Work out the finished part from the listing and answer in its coordinate system (mm). A direction names the side the tool comes from. Round coordinates to 2 decimals unless told otherwise and drop trailing zeros. Loops run counter-clockwise (first coordinate to the right, second up) from the corner with the lowest first, then second, coordinate; pieces in that order, holes last. Notation, with made-up numbers: (-9.75, 21.5) -> (33.25, 21.5) arc R22 cw to (33.25, 50.5) -> close; hole circle Ø1 at (60.25, 5). An arc over 180 degrees is marked (long way). Use one line per item in the form item = value.
```python
from build123d import *

# Parameters (mm, degrees)
BOSS_EXTRUDE1_DEPTH = 15
BOSS_EXTRUDE2_REACH = 43.075
SKETCH3_R           = 3.25
CUT_EXTRUDE1_DEPTH  = 42.075053256
FILLET1_R           = 1
FILLET2_R           = 1


with BuildPart() as part:
    # Sketch1 → Boss-Extrude1 (new, symmetric)
    with BuildSketch(Plane.XY):
        with BuildLine():
            Line((-22.5, 0), (-35, 0))
            Line((-35, 0), (-35, 3))
            Line((-35, 3), (-25.322914524, 3))
            ThreePointArc((-25.322914524, 3), (0, 25.5), (25.322914524, 3))
            Line((25.322914524, 3), (35, 3))
            Line((35, 3), (35, 0))
            Line((35, 0), (22.5, 0))
            ThreePointArc((22.5, 0), (0, 22.5), (-22.5, 0))
        make_face()
    extrude(amount=BOSS_EXTRUDE1_DEPTH, both=True)

    # Sketch2 → Boss-Extrude2 (add, up to next)
    with BuildSketch(Plane(origin=(0, 15.4, 0), x_dir=(1, 0, 0), z_dir=(0, 1, 0)), mode=Mode.PRIVATE) as boss_extrude2_sk1:
        with BuildLine():
            Line((-20.12, 6), (-20.12, -6))
            Line((-20.12, -6), (-29, -6))
            ThreePointArc((-29, -6), (-35, 0), (-29, 6))
            Line((-29, 6), (-20.12, 6))
        make_face()
    boss_extrude2_tool1 = extrude(boss_extrude2_sk1.sketch, amount=-BOSS_EXTRUDE2_REACH, mode=Mode.PRIVATE) - part.part
    boss_extrude2 = boss_extrude2_tool1.solids().sort_by_distance((-26.982165, 15.4, 0))[0]
    add(boss_extrude2)

    # Sketch3 → Cut-Extrude1 (cut, through all)
    with BuildSketch(Plane(origin=(0, 15.4, 0), x_dir=(1, 0, 0), z_dir=(0, 1, 0))):
        with Locations(Location((-29, 0, 0), (0, 0, 180))):
            Circle(SKETCH3_R)
    cut_extrude1 = extrude(amount=-CUT_EXTRUDE1_DEPTH, mode=Mode.SUBTRACT)

    # Mirror1: Boss-Extrude2, Cut-Extrude1 across plane
    add(boss_extrude2.mirror(Plane(origin=(0, 0, 0), x_dir=(0, 0, 1), z_dir=(1, 0, 0))))
    add(cut_extrude1.mirror(Plane(origin=(0, 0, 0), x_dir=(0, 0, 1), z_dir=(1, 0, 0))), mode=Mode.SUBTRACT)

    # Fillet1
    fillet1_edges = [part.edges().sort_by_distance(p)[0] for p in [
        (23.65088269, 9.533401701, -6),
        (23.65088269, 9.533401701, 6),
        (20.324615618, 15.4, 0),
    ]]
    fillet(fillet1_edges, radius=FILLET1_R)

    # Fillet2
    fillet2_edges = [part.edges().sort_by_distance(p)[0] for p in [
        (-23.65088269, 9.533401701, -6),
        (-23.65088269, 9.533401701, 6),
        (-20.324615618, 15.4, 0),
    ]]
    fillet(fillet2_edges, radius=FILLET2_R)


solid = part.part
```
(1) Find section B-B, the plane z = -1.5. Write down the section's boundary in (x, y).
Completed:
outline = (-35, 0) -> (-31.88, 0) -> (-31.88, 15.4) -> (-34.81, 15.4) -> (-34.81, 3) -> (-35, 3) -> close; (-26.12, 0) -> (-22.5, 0) arc R22.5 cw to (22.5, 0) -> (26.12, 0) -> (26.12, 15.4) -> (20.82, 15.4) arc R1 cw to (20.03, 15.78) arc R25.5 ccw to (-20.03, 15.78) arc R1 cw to (-20.82, 15.4) -> (-26.12, 15.4) -> close; (31.88, 0) -> (35, 0) -> (35, 3) -> (34.81, 3) -> (34.81, 15.4) -> (31.88, 15.4) -> close
(2) For faces 1 (the flat face through (-26, 11, -6)), 2 (the flat face through (-27, 11, 6)), 3 (the flat face through (-25, 15.4, 0)), 4 (the flat face through (30, 3, -11)), 5 (the cylindrical face through (-0.519, 25.495, 0.21)), determine the directions among +Z, -Z, +X, -X, +Y, -Y from which every point of the face is accessible in a straight line to the end or side of a thin tool.
Completed:
face_1 = -Z, -X, +Y
face_2 = +Z, -X, +Y
face_3 = +Z, -Z, -X, +Y
face_4 = -Z, +X, +Y
face_5 = +Y
(3) Consider L1, parallel to Z at x = 29, y = 4.25; L2, parallel to Y at x = -0.5, z = -0.5; L3, parallel to X at y = 17.5, z = -6. Determine where each line is inside the solid, lowest interval first.
Completed:
L1 = -6 to -3.25, 3.25 to 6
L2 = 22.49 to 25.5
L3 = -18.55 to -14.14, 14.14 to 18.55
(4) Find section C-C, the plane y = 14. State how many separate pieces and enclosed holes the cut face has, then the cut area to 3 significant figures.
Completed:
separate_pieces = 2
enclosed_holes = 2
area = 454 mm2
(5) Given P1, Ø7.5, axis at x = 29.5, z = 4, coming from the +Y side; P2, Ø2, axis at x = -21, z = 11, coming from the +Y side; P3, Ø3, axis at x = -29, z = 9, coming from the +Y side; P4, Ø4, axis at x = 29, z = 0, coming from the -Y side, each flat-ended and moving along its own axis, determine where each tip first touches the part or whether it passes through.
Completed:
P1 = 15.4
P2 = 15.82
P3 = 3
P4 = through
(6) Find section D-D, the plane x = 0. Write down the section's boundary in (y, z), then the cut area to 3 significant figures.
Completed:
outline = (22.5, -15) -> (25.5, -15) -> (25.5, 15) -> (22.5, 15) -> close
area = 90.0 mm2
(7) Find section A-A, the plane x = 27. Write down the section's boundary in (y, z), then the cut area to 3 significant figures.
Completed:
outline = (0, -15) -> (3, -15) -> (3, -6) -> (15.4, -6) -> (15.4, -2.56) -> (0, -2.56) -> close; (0, 2.56) -> (15.4, 2.56) -> (15.4, 6) -> (3, 6) -> (3, 15) -> (0, 15) -> close
area = 160 mm2
(8) For a pull along X with two mould halves and no side action, classify faces 6 (the cylindrical face through (32.002, 7.808, -1.245)), 7 (the cylindrical face through (-35, 9, 0)), 8 (the cylindrical face through (0.495, 22.495, 0.21)), 9 (the flat face through (25, 15.4, 0)) as +X half, -X half, draft (parallel to the pull), parting line (faces both ways), or undercut.
Completed:
face_6 = undercut
face_7 = -X half
face_8 = undercut
face_9 = draft
